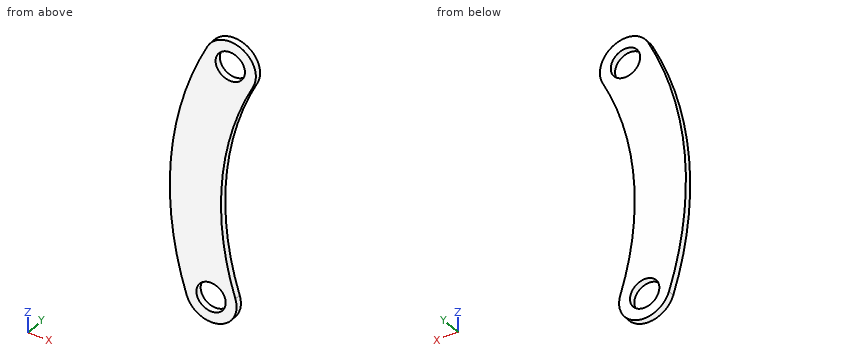
```python
from build123d import *

# Parameters (mm, degrees)
SKETCH1_R           = 6
BOSS_EXTRUDE1_DEPTH = 3
SCALE1_SCALE        = 0.225
CUT_EXTRUDE2_REACH  = 2.675
SKETCH3_R           = 1.55


with BuildPart() as part:
    # Sketch1 → Boss-Extrude1 (new body)
    with BuildSketch(Plane(origin=(0, 0, 0), x_dir=(1, 0, 0), z_dir=(0, 1, 0))):
        with BuildLine():
            ThreePointArc((-154.074297715, 50.051081743), (-161.4998099, -12.720511087), (-144.338440027, -73.555521415))
            ThreePointArc((-144.338440027, -73.555521415), (-128.198146587, -78.798700571), (-122.95496743, -62.658407131))
            ThreePointArc((-122.95496743, -62.658407131), (-137.573912137, -10.835990926), (-131.248475831, 42.63610667))
            ThreePointArc((-131.248475831, 42.63610667), (-138.953899237, 57.756505148), (-154.074297715, 50.051081743))
        make_face()
        with Locations((-142.661386773, 46.343594206)):
            Circle(SKETCH1_R, mode=Mode.SUBTRACT)
        with Locations((-133.646703729, -68.106964273)):
            Circle(SKETCH1_R, mode=Mode.SUBTRACT)
    extrude(amount=BOSS_EXTRUDE1_DEPTH)


with BuildPart() as part_1:
    # Scale1: scaled about (-145.162315364, 1.5, 11.433690498)
    add(part.part.scale(SCALE1_SCALE).moved(Location((-112.500794407, 1.1625, 8.861110136))))

    # Sketch3 → Cut-Extrude2 (cut, up to next)
    with BuildSketch(Plane(origin=(0, 1.8375, 0), x_dir=(1, 0, 0), z_dir=(0, 1, 0)), mode=Mode.PRIVATE) as cut_extrude2_sk1:
        with Locations((-144.599606431, 1.56619856)):
            Circle(SKETCH3_R)
    cut_extrude2_tool1 = extrude(cut_extrude2_sk1.sketch, amount=-CUT_EXTRUDE2_REACH, mode=Mode.PRIVATE) & part_1.part
    add(cut_extrude2_tool1.solids().sort_by_distance((-144.599606, 1.8375, -1.566199))[0], mode=Mode.SUBTRACT)
    # Sketch3 → Cut-Extrude2 (cut, up to next)
    with BuildSketch(Plane(origin=(0, 1.8375, 0), x_dir=(1, 0, 0), z_dir=(0, 1, 0)), mode=Mode.PRIVATE) as cut_extrude2_sk2:
        with Locations((-142.571302746, -24.185177098)):
            Circle(SKETCH3_R)
    cut_extrude2_tool2 = extrude(cut_extrude2_sk2.sketch, amount=-CUT_EXTRUDE2_REACH, mode=Mode.PRIVATE) & part_1.part
    add(cut_extrude2_tool2.solids().sort_by_distance((-142.571303, 1.8375, 24.185177))[0], mode=Mode.SUBTRACT)


solid = part_1.part
```
Check sheet for the modelled part. Datum: model origin and axes. Units: mm. Round coordinates to 2 decimals unless told otherwise and drop trailing zeros. Order: outer loops, then holes, each group sorted by start corner. A loop starts at its lowest first (then second) coordinate and runs counter-clockwise, first axis right, second up. Notation, with made-up numbers: (37.5, 88.25) - (82.5, 88.25) arc R23 cw to (82.5, 105.25) - close; hole circle Ø4 at (29.5, 24.25). An arc over 180 degrees is marked (long way). Write item = value, one per line.
Q1. Section check C-C (z = -1). Record the boundary of the cut face in (x, y), and give its area (3 significant figures).
Computed:
outline = (-147.59, 1.16) - (-146.04, 1.16) - (-146.04, 1.84) - (-147.59, 1.84) - close; (-143.16, 1.16) - (-141.96, 1.16) - (-141.96, 1.84) - (-143.16, 1.84) - close
area = 1.85 mm^2
Q2. Thickness scan on line 1 along Z through (x, y) = (-146, 1.7); line 2 along Z through (x, y) = (-145.75, 1.2) (3 decimals); line 3 along X through (y, z) = (1.6, 7.5). Record the ranges inside material, lowest first.
Computed:
line_1 = -3.87 to -2.23, -0.9 to 23.23
line_2 = -4.009 to -2.605, -0.527 to 23.797
line_3 = -148.93 to -143.52
Q3. Section check D-D (x = -145.75). Record the boundary of the cut face in (y, z) (1 decimal), and give its area (3 significant figures).
Computed:
outline = (1.2, -4) - (1.8, -4) - (1.8, -2.6) - (1.2, -2.6) - close; (1.2, -0.5) - (1.8, -0.5) - (1.8, 23.8) - (1.2, 23.8) - close
area = 17.4 mm^2
Q4. Section check B-B (y = 1.4). Record the boundary of the cut face in (x, z).
Computed:
outline = (-147.17, -2.4) arc R2.7 ccw to (-142.03, -0.73) arc R31.05 cw to (-140.17, 22.96) arc R2.7 ccw to (-144.98, 25.41) arc R36.45 ccw to start; hole circle Ø3.1 at (-144.6, -1.57); hole circle Ø3.1 at (-142.57, 24.19)
Q5. Section check A-A (x = -142.5). Record the boundary of the cut face in (y, z).
Computed:
outline = (1.16, -3.26) - (1.84, -3.26) - (1.84, 0.85) - (1.16, 0.85) - close; (1.16, 16.87) - (1.84, 16.87) - (1.84, 22.64) - (1.16, 22.64) - close; (1.16, 25.73) - (1.84, 25.73) - (1.84, 26.88) - (1.16, 26.88) - close
Q6. Go/stop test with a flat-tipped pin: pin 1 (5 mm diameter, centred on x = -142.57, z = 24.19, fed in from -Y). Record where the tip stops, or that it passes through.
Computed:
pin_1 = 1.16
